```python
from build123d import *

# Parameters (mm, degrees)
SKETCH1_R                       = 35
BOSS_EXTRUDE1_DEPTH             = 40
SKETCH2_R                       = 5
BOSS_EXTRUDE2_DEPTH             = 22
BOSS_EXTRUDE3_DEPTH             = 5
HOLE1_D                         = 50
BOSS_EXTRUDE4_REACH             = 106.523
SKETCH7_W                       = 75
SKETCH7_H                       = 25
BOSS_EXTRUDE4_DIRECTION_2_REACH = 106.523
HOLE2_D                         = 50
CUT_EXTRUDE1_DEPTH              = 106.386194542
CUT_EXTRUDE1_DEPTH_BACK         = 106.386194542
SKETCH11_W                      = 24
SKETCH11_H                      = 40
HOLE3_D                         = 8
FILLET1_R                       = 5


with BuildPart() as part:
    # Sketch1 → Boss-Extrude1 (new, symmetric)
    with BuildSketch(Plane.XY):
        Circle(SKETCH1_R)
    extrude(amount=BOSS_EXTRUDE1_DEPTH, both=True)

    # Sketch2 → Boss-Extrude2 (add, symmetric)
    with BuildSketch(Plane.XY):
        with BuildLine():
            Line((-33.732608688, 9.333333333), (-14.456832295, 79))
            ThreePointArc((-14.456832295, 79), (0, 90), (14.456832295, 79))
            Line((14.456832295, 79), (33.732608688, 9.333333333))
            ThreePointArc((33.732608688, 9.333333333), (0, 35), (-33.732608688, 9.333333333))
        make_face()
        with Locations((0, 75)):
            Circle(SKETCH2_R, mode=Mode.SUBTRACT)
    extrude(amount=BOSS_EXTRUDE2_DEPTH, both=True)

    # Sketch3 → Boss-Extrude3 (add, symmetric)
    with BuildSketch(Plane(origin=(0, 0, 0), x_dir=(0, 0, -1), z_dir=(1, 0, 0))):
        Polygon((-40, 35), (-22, 59), (22, 59), (40, 35), (40, 0), (-40, 0), align=None)
    extrude(amount=BOSS_EXTRUDE3_DEPTH, both=True)

    # Hole1 (through all)
    with Locations(Plane.XY.offset(40)):
        with Locations((0, 0)):
            Hole(HOLE1_D / 2)

    # Boss-Extrude4: up to this face of the body (flat: up to its plane)
    boss_extrude4_end = Plane(part.part.faces().sort_by_distance((0, -34.010050506, -40))[0])
    # Sketch7 → Boss-Extrude4 (add, up to the picked face)
    with BuildSketch(Plane.XY, mode=Mode.PRIVATE) as boss_extrude4_sk1:
        Rectangle(SKETCH7_W, SKETCH7_H)
    boss_extrude4_tool1 = split(extrude(boss_extrude4_sk1.sketch, amount=-BOSS_EXTRUDE4_REACH, mode=Mode.PRIVATE), bisect_by=boss_extrude4_end, keep=Keep.BOTH, mode=Mode.PRIVATE)
    add(boss_extrude4_tool1.solids().sort_by(Axis((0, 0, 0), (0, 0, -1)))[0])

    # Boss-Extrude4 direction 2: up to this face of the body (flat: up to its plane)
    boss_extrude4_direction_2_end = Plane(part.part.faces().sort_by_distance((0, -34.010050506, 40))[0])
    # Sketch7 → Boss-Extrude4 direction 2 (add, up to the picked face)
    with BuildSketch(Plane.XY, mode=Mode.PRIVATE) as boss_extrude4_direction_2_sk1:
        Rectangle(SKETCH7_W, SKETCH7_H)
    boss_extrude4_direction_2_tool1 = split(extrude(boss_extrude4_direction_2_sk1.sketch, amount=BOSS_EXTRUDE4_DIRECTION_2_REACH, mode=Mode.PRIVATE), bisect_by=boss_extrude4_direction_2_end, keep=Keep.BOTH, mode=Mode.PRIVATE)
    add(boss_extrude4_direction_2_tool1.solids().sort_by(Axis((0, 0, 0), (0, 0, 1)))[0])

    # Hole2 (through all)
    with Locations(Plane.XY.offset(40)):
        with Locations((0, 0)):
            Hole(HOLE2_D / 2)

    # Sketch11 → Cut-Extrude1 (cut, two sides: drawn at the far end of the back side and taken through both)
    with BuildSketch(Plane(origin=(0, 0, 0), x_dir=(0, 0, -1), z_dir=(1, 0, 0)).offset(-CUT_EXTRUDE1_DEPTH_BACK)):
        with Locations((0, 70)):
            Rectangle(SKETCH11_W, SKETCH11_H)
    extrude(amount=CUT_EXTRUDE1_DEPTH + CUT_EXTRUDE1_DEPTH_BACK, mode=Mode.SUBTRACT)

    # Hole3 (through all)
    with Locations(Plane(origin=(37.5, 0, 0), x_dir=(0, 0, -1), z_dir=(1, 0, 0))):
        with Locations((-25, 0), (25, 0)):
            Hole(HOLE3_D / 2)

    # Fillet1
    fillet1_edges = [part.edges().sort_by_distance(p)[0] for p in [
        (-32.691742077, 12.5, 31),
    ]]
    fillet(fillet1_edges, radius=FILLET1_R - 0.0001)  # a hair under: the kernel refuses the full size
    fillet1_2_edges = [part.edges().sort_by_distance(p)[0] for p in [
        (32.691742077, 12.5, 31),
    ]]
    fillet(fillet1_2_edges, radius=FILLET1_R)
    fillet1_3_edges = [part.edges().sort_by_distance(p)[0] for p in [
        (-32.691742077, -12.5, 0),
    ]]
    fillet(fillet1_3_edges, radius=FILLET1_R)
    fillet1_4_edges = [part.edges().sort_by_distance(p)[0] for p in [
        (32.691742077, -12.5, 0),
    ]]
    fillet(fillet1_4_edges, radius=FILLET1_R)


solid = part.part
```
Geometry: final body of the model. Coordinates: model frame, mm. A direction names the side the tool comes from. Give positions to 0.01 mm unless a question says otherwise; leave off trailing zeros. Write each loop counter-clockwise with the first axis right and the second up, starting at its lowest first coordinate (ties: lowest second). Pieces come first, ordered by that corner, then holes.
1. Section query A-A, the plane y = 0. Return loops of the section in (x, z).
2. Section query D-D, the plane y = 73. Return loops of the section in (x, z).
3. Line query: probe 1 along Y at (x, z) = (0, -16); probe 2 along Z at (x, y) = (29.75, 0); probe 3 along Z at (x, y) = (-8, 84.5). Output: solid intervals per line, ascending.
4. Section query B-B, the plane z = 25. Return loops of the section in (x, y), then the cut area to 3 significant figures.
5. Pin query (flat end, axial travel): P1, Ø20, axis at x = 3.5, y = 75, coming from the +Z side; P2, Ø12, axis at x = -12.5, z = 25, coming from the -Y side; P3, Ø13, axis at x = 0, y = 75, coming from the -Z side. Return the tip coordinate at first contact, or that it passes through.
6. Draft query along Y for faces 4 (the flat face through (0, 61, 22)), 5 (the cylindrical face through (-1.08, 70.12, -17.07)), 6 (the cylindrical face through (-31.2, -2.4, 21.8)), 7 (the cylindrical face through (-20.446, 28.407, 31.126)). Return one class per face: released by +Y, released by -Y, zero draft, split by the parting line, or undercut.
7. Reachability of faces 1 (the flat face through (0, 65, 12)), 2 (the cylindrical face through (21, 28, -31)), 3 (the flat face through (5, 44, 29)) from +Z, -Z, +X, -X, +Y, -Y: full face, straight path, thin tool, end or side. Return the list, or none.
8. Section query C-C, the plane x = 0. Return loops of the section in (y, z), then the cut area to 3 significant figures.
Computed:
1. outline: (-37.5, -40) - (-25, -40) - (-25, -29) - (-37.5, -29) - close; (-37.5, -21) - (-25, -21) - (-25, 21) - (-37.5, 21) - close; (-37.5, 29) - (-25, 29) - (-25, 40) - (-37.5, 40) - close; (25, -40) - (37.5, -40) - (37.5, -29) - (25, -29) - close; (25, -21) - (37.5, -21) - (37.5, 21) - (25, 21) - close; (25, 29) - (37.5, 29) - (37.5, 40) - (25, 40) - close
2. outline: (-16.12, -22) - (-4.58, -22) - (-4.58, -12) - (-16.12, -12) - close; (-16.12, 12) - (-4.58, 12) - (-4.58, 22) - (-16.12, 22) - close; (4.58, -22) - (16.12, -22) - (16.12, -12) - (4.58, -12) - close; (4.58, 12) - (16.12, 12) - (16.12, 22) - (4.58, 22) - close
3. probe 1: y = -35 to -25, 25 to 70, 80 to 90
3. probe 2: z = -40 to -29, -21 to 21, 29 to 40
3. probe 3: z = -22 to -12, 12 to 22
4. outline: (-37.5, -12.5) - (-35.97, -12.5) arc R5 cw to (-31.47, -15.31) arc R35 ccw to (31.47, -15.31) arc R5 cw to (35.97, -12.5) - (37.5, -12.5) - (37.5, -4) - (24.68, -4) arc R25 cw to (-24.68, -4) - (-37.5, -4) - close; (-37.5, 4) - (-24.68, 4) arc R25 cw to (24.68, 4) - (37.5, 4) - (37.5, 12.5) - (35.97, 12.5) arc R5 cw to (31.47, 15.31) arc R35 ccw to (5, 34.64) - (5, 55) - (-5, 55) - (-5, 34.64) arc R35 ccw to (-31.47, 15.31) arc R5 cw to (-35.97, 12.5) - (-37.5, 12.5) - close
4. area: 2,050 mm2
5. P1: stops at z = 22
5. P2: stops at y = -34.39
5. P3: stops at z = -22
6. face 4: zero draft
6. face 5: undercut
6. face 6: undercut
6. face 7: released by +Y
7. face 1: +X, -X, +Y
7. face 2: -Z, +X, +Y
7. face 3: +Z, +X, +Y
8. outline: (-35, -40) - (-25, -40) - (-25, 40) - (-35, 40) - close; (25, -40) - (35, -40) - (59, -22) - (70, -22) - (70, -12) - (50, -12) - (50, 12) - (70, 12) - (70, 22) - (59, 22) - (35, 40) - (25, 40) - close; (80, -22) - (90, -22) - (90, -12) - (80, -12) - close; (80, 12) - (90, 12) - (90, 22) - (80, 22) - close
8. area: 3,290 mm2
